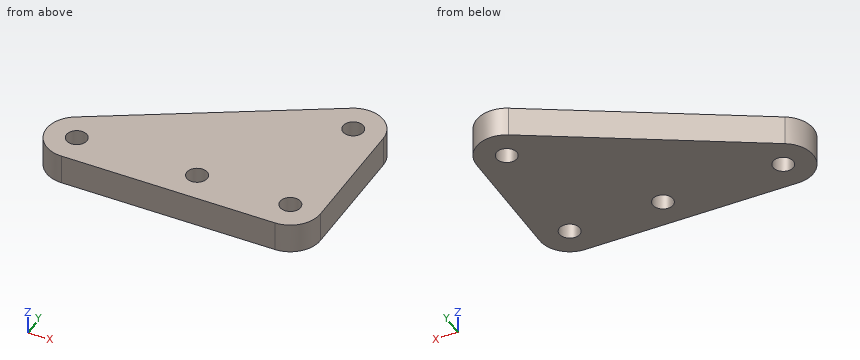
from build123d import *

# Parameters (mm, degrees)
SKETCH_1_R      = 1.7
EXTRUDE_1_DEPTH = 5


with BuildPart() as part:
    # ｽｹｯﾁ1 → ﾎﾞｽ - 押し出し1 (new body)
    with BuildSketch(Plane.XY):
        with BuildLine():
            ThreePointArc((35.507041555, -5), (39.042575461, -3.535533906), (40.507041555, 0))
            Line((40.507041555, 0), (40.507041555, 20.5))
            ThreePointArc((40.507041555, 20.5), (38.007041622, 24.830126981), (33.007041688, 24.830127096))
            Line((33.007041688, 24.830127096), (-2.50000007, 4.330126978))
            ThreePointArc((-2.50000007, 4.330126978), (-4.829629126, -1.294095246), (-3.8e-08, -5))
            Line((-3.8e-08, -5), (35.507041555, -5))
        make_face()
        Circle(SKETCH_1_R, mode=Mode.SUBTRACT)
        with Locations((20, 0)):
            Circle(SKETCH_1_R, mode=Mode.SUBTRACT)
        with Locations((35.507041555, 0)):
            Circle(SKETCH_1_R, mode=Mode.SUBTRACT)
        with Locations((35.507041555, 20.5)):
            Circle(SKETCH_1_R, mode=Mode.SUBTRACT)
    extrude(amount=EXTRUDE_1_DEPTH)


solid = part.part
Design review of the part built by this model. Coordinates are the model's own, in mm. Round coordinates to 2 decimals unless told otherwise and drop trailing zeros. Write each loop counter-clockwise with the first axis right and the second up, starting at its lowest first coordinate (ties: lowest second). Pieces come first, ordered by that corner, then holes. Notation, with made-up numbers: (-28.75, -11.75) - (-15.75, -11.75) arc R17 ccw to (-15.75, -5.75) - close; hole circle Ø6 at (-15, 59.5). An arc over 180 degrees is marked (long way). Use a Markdown table: item, result. Add a question column.
1. Wall thickness on probe 1 along Y at (x, z) = (35, 4.75); probe 2 along X at (y, z) = (-0.5, 4.15); probe 3 along X at (y, z) = (19.5, 2.2) (3 decimals): over which ranges is each line inside the solid? List them lowest first.
2. We need section C-C (x = 20). State the section outline as (y, z) points, then the cut area to 3 significant figures.
3. We need section B-B (y = -0.5). State the section outline as (x, z) points, then the cut area to 3 significant figures.
4. Clearance check with flat-ended pins moving along their axes: pin 1 (5.5 mm diameter, centred on x = 35.51, y = 20.5, fed in from -Z); pin 2 (1.5 mm diameter, centred on y = 14.5, z = 3.5, fed in from -X); pin 3 (2 mm diameter, centred on x = 27.5, z = 2, fed in from +Y). State where each tip first meets the part, or that it passes through.
5. We need section A-A (z = 3.5). State the section outline as (x, y) points.
6. We need section D-D (y = 9). State the section outline as (x, z) points.
Output:
| question | item | result |
|---|---|---|
| 1 | probe 1 | y = -5 to -1.62, 1.62 to 18.88, 22.12 to 25.47 |
| 1 | probe 2 | x = -4.97 to -1.62, 1.62 to 18.38, 21.62 to 33.88, 37.13 to 40.48 |
| 1 | probe 3 | x = 23.775 to 34.132, 36.882 to 40.507 |
| 2 | outline | (-5, 0) - (-1.7, 0) - (-1.7, 5) - (-5, 5) - close; (1.7, 0) - (17.32, 0) - (17.32, 5) - (1.7, 5) - close |
| 2 | area | 94.6 mm2 |
| 3 | outline | (-4.97, 0) - (-1.62, 0) - (-1.62, 5) - (-4.97, 5) - close; (1.62, 0) - (18.38, 0) - (18.38, 5) - (1.62, 5) - close; (21.62, 0) - (33.88, 0) - (33.88, 5) - (21.62, 5) - close; (37.13, 0) - (40.48, 0) - (40.48, 5) - (37.13, 5) - close |
| 3 | area | 179 mm2 |
| 4 | pin 1 | stops at z = 0 |
| 4 | pin 2 | stops at x = 13.82 |
| 4 | pin 3 | stops at y = 22.23 |
| 5 | outline | (-2.5, 4.33) arc R5 ccw to (0, -5) - (35.51, -5) arc R5 ccw to (40.51, 0) - (40.51, 20.5) arc R5 ccw to (33.01, 24.83) - close; hole circle Ø3.4 at (0, 0); hole circle Ø3.4 at (20, 0); hole circle Ø3.4 at (35.51, 0); hole circle Ø3.4 at (35.51, 20.5) |
| 6 | outline | (5.59, 0) - (40.51, 0) - (40.51, 5) - (5.59, 5) - close |
